from build123d import *

# Parameters (mm, degrees)
SKETCH_1_R      = 12.4
SKETCH_1_R_2    = 1.7
EXTRUDE_1_DEPTH = 5
SKETCH_2_R      = 13.9
SKETCH_2_R_2    = 12.4
EXTRUDE_2_DEPTH = 0.5


with BuildPart() as part:
    # 草图1 → 凸台-拉伸1 (new body)
    with BuildSketch(Plane.XY):
        Circle(SKETCH_1_R)
        with Locations((-6.5, 0)):
            Circle(SKETCH_1_R_2, mode=Mode.SUBTRACT)
        with Locations((6.5, 0)):
            Circle(SKETCH_1_R_2, mode=Mode.SUBTRACT)
    extrude(amount=EXTRUDE_1_DEPTH)

    # 草图2 → 凸台-拉伸2 (add)
    with BuildSketch(Plane.XY):
        Circle(SKETCH_2_R)
        Circle(SKETCH_2_R_2, mode=Mode.SUBTRACT)
    extrude(amount=EXTRUDE_2_DEPTH)


solid = part.part
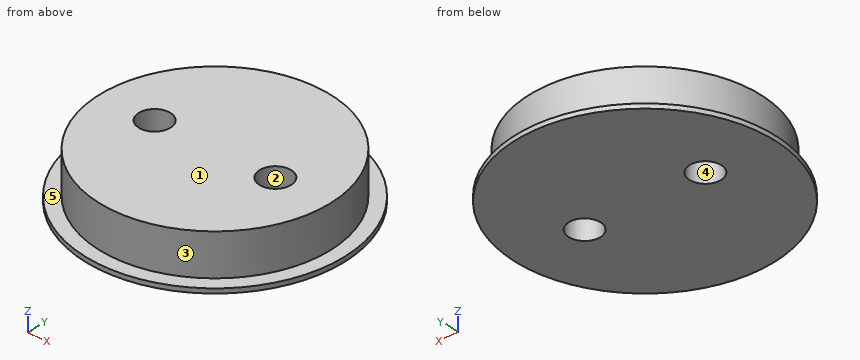
The listing builds one solid part. Answer for the finished solid, in the listing's coordinates (mm). Face numbers are marked on the shaded views. A direction names the side the tool comes from. Coordinates: 2 decimals unless noted, no trailing zeros. Write each loop counter-clockwise with the first axis right and the second up, starting at its lowest first coordinate (ties: lowest second). Pieces come first, ordered by that corner, then holes. Notation, with made-up numbers: M -31.75,-10 L -14.75,-10 A14 ccw -14.75,3 Z; hole C 69,58.25 d2. An arc over 180 degrees is marked long. Put each result on its own line as item: value. Start each with the question number.
1. A cutting plane is placed at B-B on y = 0. Write down the section's boundary in (x, z).
2. A cutting plane is placed at C-C on x = -6.5. Write down the section's boundary in (y, z), then the cut area to 3 significant figures.
3. Flat-ended cylindrical pins translate along their axes: P1, Ø2, axis at y = -10.5, z = 3, coming from the -X side; P2, Ø1, axis at x = -4.5, z = 4, coming from the +Y side; P3, Ø2, axis at y = 6, z = 4, coming from the +X side. Find the tip coordinate at first contact, or state that the pin passes through.
4. Consider line 1 (Z direction, x = 5.5, y = -12); line 2 (X direction, y = 1, z = 4.4); line 3 (Y direction, x = -6.5, z = 1.8). Determine where each line is inside the solid, lowest interval first. Write a range as from..to.
5. Which of the six approach directions +Z, -Z, +X, -X, +Y, -Y give full straight-line access (tool end or side, diameter ignored) to the marked faces 4 and 5?
6. A cutting plane is placed at D-D on z = 4.55. Write down the section's boundary in (x, y), then the cut area to 3 significant figures.
7. For a pull along Y with two mould halves and no side action, classify the marked faces 1, 2 and 3 as pulls with the +Y half, pulls with the -Y half, needs draft (parallel to the pull), parting line crosses it, or undercut.
8. A cutting plane is placed at A-A on x = 0. Write down the section's boundary in (y, z), then the cut area to 4 significant figures.
Resolved:
1. outline: M -13.9,0 L -8.2,0 L -8.2,5 L -12.4,5 L -12.4,0.5 L -13.9,0.5 Z; M -4.8,0 L 4.8,0 L 4.8,5 L -4.8,5 Z; M 8.2,0 L 13.9,0 L 13.9,0.5 L 12.4,0.5 L 12.4,5 L 8.2,5 Z
2. outline: M -12.29,0 L -1.7,0 L -1.7,5 L -10.56,5 L -10.56,0.5 L -12.29,0.5 Z; M 1.7,0 L 12.29,0 L 12.29,0.5 L 10.56,0.5 L 10.56,5 L 1.7,5 Z
2. area: 90.3 mm2
3. P1: stops at x = -7.97
3. P2: stops at y = 11.74
3. P3: stops at x = 11.35
4. line 1: z = 0..0.5
4. line 2: x = -12.36..-7.87, -5.13..5.13, 7.87..12.36
4. line 3: y = -10.56..-1.7, 1.7..10.56
5. face 4: +Z, -Z
5. face 5: +Z
6. outline: C 0,0 d24.8; hole C -6.5,0 d3.4; hole C 6.5,0 d3.4
6. area: 465 mm2
7. face 1: needs draft
7. face 2: undercut
7. face 3: parting line crosses it
8. outline: M -13.9,0 L 13.9,0 L 13.9,0.5 L 12.4,0.5 L 12.4,5 L -12.4,5 L -12.4,0.5 L -13.9,0.5 Z
8. area: 125.5 mm2
